The listing builds one solid part. Answer for the finished solid, in the listing's coordinates (mm). Give positions to 0.01 mm unless a question says otherwise; leave off trailing zeros. Write each loop counter-clockwise with the first axis right and the second up, starting at its lowest first coordinate (ties: lowest second). Pieces come first, ordered by that corner, then holes.
```python
from build123d import *

# Parameters (mm, degrees)
SKETCH_1_R      = 1.5
SKETCH_1_R_2    = 10.5
SKETCH_1_W      = 10
SKETCH_1_H      = 6
SKETCH_1_W_2    = 8
SKETCH_1_H_2    = 14.5
SKETCH_1_W_3    = 23
SKETCH_1_H_3    = 19.5
EXTRUDE_1_DEPTH = 6


with BuildPart() as part:
    # Эскиз1 → Бобышка-Вытянуть1 (new body)
    with BuildSketch(Plane.XY):
        Polygon((-126.5, 22), (-126.5, 10.5), (-132.5, 10.5), (-132.5, -4.5), (-126.5, -4.5), (-126.5, -13.9), (-120.5, -13.9), (-120.5, -22), (120.5, -22), (120.5, -13.9), (126.5, -13.9), (126.5, -4.5), (132.5, -4.5), (132.5, 10.5), (126.5, 10.5), (126.5, 22), align=None)
        with Locations((57.5, 17)):
            Circle(SKETCH_1_R, mode=Mode.SUBTRACT)
        with Locations((110, 3)):
            Circle(SKETCH_1_R_2, mode=Mode.SUBTRACT)
        with Locations((57.5, -17)):
            Circle(SKETCH_1_R, mode=Mode.SUBTRACT)
        with Locations((-57.5, 17)):
            Circle(SKETCH_1_R, mode=Mode.SUBTRACT)
        with Locations((-110, 3)):
            Circle(SKETCH_1_R_2, mode=Mode.SUBTRACT)
        with Locations((-57.5, -17)):
            Circle(SKETCH_1_R, mode=Mode.SUBTRACT)
        with Locations((33, 17)):
            Rectangle(SKETCH_1_W, SKETCH_1_H, mode=Mode.SUBTRACT)
        with Locations((82, 17)):
            Rectangle(SKETCH_1_W, SKETCH_1_H, mode=Mode.SUBTRACT)
        with Locations((33, -17)):
            Rectangle(SKETCH_1_W, SKETCH_1_H, mode=Mode.SUBTRACT)
        with Locations((82, -17)):
            Rectangle(SKETCH_1_W, SKETCH_1_H, mode=Mode.SUBTRACT)
        with Locations((-33, 17)):
            Rectangle(SKETCH_1_W, SKETCH_1_H, mode=Mode.SUBTRACT)
        with Locations((-82, 17)):
            Rectangle(SKETCH_1_W, SKETCH_1_H, mode=Mode.SUBTRACT)
        with Locations((-33, -17)):
            Rectangle(SKETCH_1_W, SKETCH_1_H, mode=Mode.SUBTRACT)
        with Locations((-82, -17)):
            Rectangle(SKETCH_1_W, SKETCH_1_H, mode=Mode.SUBTRACT)
        with Locations((-22.5, 6.749994)):
            Rectangle(SKETCH_1_W_2, SKETCH_1_H_2, mode=Mode.SUBTRACT)
        with Locations((2e-06, 4.249994)):
            Rectangle(SKETCH_1_W_3, SKETCH_1_H_3, mode=Mode.SUBTRACT)
    extrude(amount=EXTRUDE_1_DEPTH)


solid = part.part
```
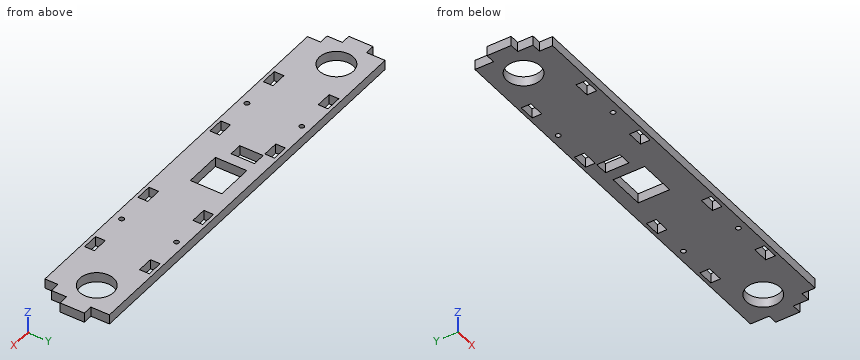
Item 1: A cutting plane is placed at B-B, the plane z = 2.6. Count the separate pieces of the cut face and the enclosed holes in it, plus the area to 3 significant figures.
Conclusion:
separate pieces: 1
enclosed holes: 16
area: 9,450 mm2
Item 2: A cutting plane is placed at A-A, the plane x = 110. Give the vertices of the cut face in (y, z).
Conclusion:
outline: (-22, 0) - (-7.5, 0) - (-7.5, 6) - (-22, 6) - close; (13.5, 0) - (22, 0) - (22, 6) - (13.5, 6) - close
Item 3: Consider probe 1 along Y at (x, z) = (78, 5.45); probe 2 along X at (y, z) = (19.5, 2.1); probe 3 along Y at (x, z) = (57.5, 3.45). Determine where each line is inside the solid, lowest interval first.
Conclusion:
probe 1: y = -22 to -20, -14 to 14, 20 to 22
probe 2: x = -126.5 to -87, -77 to -38, -28 to 28, 38 to 77, 87 to 126.5
probe 3: y = -22 to -18.5, -15.5 to 15.5, 18.5 to 22
Item 4: Each of these flat-tipped pins is pushed along its axis until it touches: P1, Ø1.8, axis at y = 16, z = 3, coming from the -X side; P2, Ø3, axis at y = -15.5, z = 3.5, coming from the +X side; P3, Ø3, axis at x = 128.5, z = 4, coming from the +Y side. Where does it stop, or does it pass through?
Conclusion:
P1: stops at x = -126.5
P2: stops at x = 120.5
P3: stops at y = 10.5
